from build123d import *

# Parameters (mm, degrees)
F0_W     = 6
F0_H     = 22
F1_DEPTH = 5
F3_DEPTH = 6
F5_D     = 3.3
F7_D     = 4.4


with BuildPart() as f1:
    # F0 (on Top) → F1 (new body)
    with BuildSketch(Plane.XY):
        with Locations((-2.4757032864, -3.9350604638)):
            Rectangle(F0_W, F0_H)
    extrude(amount=F1_DEPTH)

    # F2 (on face) → F3 (join)
    with BuildSketch(Plane(origin=(-5.4757032864, 0, 0), x_dir=(0, -1, 0), z_dir=(-1, 0, 0))):
        Polygon((-10.0649395362, 0), (-7.0649395362, 0), (-7.0649395362, 5), (-7.0649395362, 33), (-10.0649395362, 33), align=None)
    extrude(amount=-F3_DEPTH)

    # F5 (through all)
    with Locations(Plane.XY.offset(5)):
        with Locations((-2.4757032864, -11.6850604638)):
            Hole(F5_D / 2)

    # F7 (through all)
    with Locations(Plane.XZ.offset(-7.0649395362)):
        with Locations((-2.4757032864, 27.8)):
            Hole(F7_D / 2)


solid = f1.part
Read the model definition and answer for the solid it produces. Units are mm, in the model's axes. A direction names the side the tool comes from. Round coordinates to 2 decimals unless told otherwise and drop trailing zeros. Write each loop counter-clockwise with the first axis right and the second up, starting at its lowest first coordinate (ties: lowest second). Pieces come first, ordered by that corner, then holes. Notation, with made-up numbers: M -35.75,78 L -3.75,78 A19 cw -3.75,102 Z; hole C 60,39 d3. An arc over 180 degrees is marked long. Use a Markdown table: item, result.
1) Flat-ended cylindrical pins translate along their axes: pin 1 (3 mm diameter, centred on x = -4, z = 22, fed in from -Y); pin 2 (10 mm diameter, centred on y = -1.5, z = 21, fed in from -X). Find the tip coordinate at first contact, or state that the pin passes through.
Answers follow:
| item | result |
|---|---|
| pin 1 | stops at y = 7.06 |
| pin 2 | passes through |
2) Straight lines are drawn through the part: line 1 along Y through (x, z) = (-1.35, 14); line 2 along Z through (x, y) = (-0.1, 3.75); line 3 along Z through (x, y) = (-3, 9). For each, find the intervals that lie inside material, in ascending order. Write a range as [from, to].
Answers follow:
| item | result |
|---|---|
| line 1 | y = [7.06, 10.06] |
| line 2 | z = [0, 5] |
| line 3 | z = [0, 25.66], [29.94, 33] |
3) The part is cut by section C-C (y = 5.5). Write down the section's boundary in (x, z).
Answers follow:
| item | result |
|---|---|
| outline | M -5.48,0 L 0.52,0 L 0.52,5 L -5.48,5 Z |
4) The part is cut by section B-B (x = -1.6). Write down the section's boundary in (y, z), plus the area to 3 significant figures.
Answers follow:
| item | result |
|---|---|
| outline | M -14.94,0 L -13.08,0 L -13.08,5 L -14.94,5 Z; M -10.29,0 L 10.06,0 L 10.06,25.78 L 7.06,25.78 L 7.06,5 L -10.29,5 Z; M 7.06,29.82 L 10.06,29.82 L 10.06,33 L 7.06,33 Z |
| area | 183 mm2 |
5) A tool of negligible diameter and unlimited length cuts with its end or side. For faces 1 (the flat face through (-3, 7.065, 19)), 2 (the cylindrical face through (-2.118, -13.296, 2.465)), from which of +Z, -Z, +X, -X, +Y, -Y can it reach the whole face along a straight path? Write none if from no direction.
Answers follow:
| item | result |
|---|---|
| face 1 | +Z, +X, -X, -Y |
| face 2 | +Z, -Z |
6) The part is cut by section A-A (z = 27.8). Write down the section's boundary in (x, y), plus the area to 3 significant figures.
Answers follow:
| item | result |
|---|---|
| outline | M -5.48,7.06 L -4.68,7.06 L -4.68,10.06 L -5.48,10.06 Z; M -0.28,7.06 L 0.52,7.06 L 0.52,10.06 L -0.28,10.06 Z |
| area | 4.80 mm2 |
7) For a pull along Z with two mould halves and no side action, classify faces 3 (the flat face through (-5.476, 2, 4)), 4 (the flat face through (-3, -4, 5)), 5 (the cylindrical face through (-4.574, 8.586, 28.461)), 6 (the flat face through (-3, -2, 0)) as pulls with the +Z half, pulls with the -Z half, needs draft (parallel to the pull), parting line crosses it, or undercut.
Answers follow:
| item | result |
|---|---|
| face 3 | needs draft |
| face 4 | pulls with the +Z half |
| face 5 | undercut |
| face 6 | pulls with the -Z half |
8) The part is cut by section D-D (z = 6.5). Write down the section's boundary in (x, y).
Answers follow:
| item | result |
|---|---|
| outline | M -5.48,7.06 L 0.52,7.06 L 0.52,10.06 L -5.48,10.06 Z |
